Geometry: final body of the model. Coordinates: model frame, mm. Give positions to 0.01 mm unless a question says otherwise; leave off trailing zeros. Write each loop counter-clockwise with the first axis right and the second up, starting at its lowest first coordinate (ties: lowest second). Pieces come first, ordered by that corner, then holes. Notation, with made-up numbers: (-8, -37) - (28, -37) arc R28 ccw to (28, -10) - close; hole circle Ø11 at (-17, 50). An arc over 180 degrees is marked (long way). One line per question, with ' | ' between items. Start each with the question number.
```python
from build123d import *

# Parameters (mm, degrees)
F1_DEPTH = 127


with BuildPart() as f1:
    # F0 (on Front) → F1 (new body)
    with BuildSketch(Plane.XZ):
        with BuildLine():
            ThreePointArc((5.4872727498, -3.1956748535), (6.130525343, -1.6550404888), (6.35, 0))
            ThreePointArc((6.35, 0), (6.136710925, 1.6319555825), (5.5111719612, 3.1542802054))
            ThreePointArc((5.5111719612, 3.1542802054), (3.1956748226, 5.4872727678), (0.0238991973, 6.3499550257))
            ThreePointArc((0.0238991973, 6.3499550257), (-3.1542802223, 5.5111719515), (-5.4872727914, 3.195674782))
            ThreePointArc((-5.4872727914, 3.195674782), (-6.3499550258, 0.0238991699), (-5.5111719612, -3.1542802054))
            ThreePointArc((-5.5111719612, -3.1542802054), (-3.1956748226, -5.4872727678), (-0.0238991973, -6.3499550257))
            ThreePointArc((-0.0238991973, -6.3499550257), (3.1542801864, -5.511171972), (5.4872727498, -3.1956748535))
        make_face()
        with BuildLine():
            ThreePointArc((5.5111719612, 3.1542802054), (6.136710925, 1.6319555825), (6.35, 0))
            ThreePointArc((6.35, 0), (6.130525343, -1.6550404888), (5.4872727498, -3.1956748535))
            Line((5.4872727498, -3.1956748535), (7.3322964871, -0.027596355))
            Line((7.3322964871, -0.027596355), (5.5111719612, 3.1542802054))
        make_face()
        with BuildLine():
            ThreePointArc((0.0238991973, 6.3499550257), (3.1956748226, 5.4872727678), (5.5111719612, 3.1542802054))
            Line((5.5111719612, 3.1542802054), (3.690047388, 6.3361568484))
            Line((3.690047388, 6.3361568484), (0.0238991973, 6.3499550257))
        make_face()
        with BuildLine():
            Line((3.6422490991, -6.3637532034), (5.4872727498, -3.1956748535))
            ThreePointArc((5.4872727498, -3.1956748535), (3.1542801864, -5.511171972), (-0.0238991973, -6.3499550257))
            Line((-0.0238991973, -6.3499550257), (3.6422490991, -6.3637532034))
        make_face()
        with BuildLine():
            ThreePointArc((-5.4872727914, 3.195674782), (-3.1542802223, 5.5111719515), (0.0238991973, 6.3499550257))
            Line((0.0238991973, 6.3499550257), (-3.6422490991, 6.3637532034))
            Line((-3.6422490991, 6.3637532034), (-5.4872727914, 3.195674782))
        make_face()
        with BuildLine():
            Line((-3.690047388, -6.3361568484), (-0.0238991973, -6.3499550257))
            ThreePointArc((-0.0238991973, -6.3499550257), (-3.1956748226, -5.4872727678), (-5.5111719612, -3.1542802054))
            Line((-5.5111719612, -3.1542802054), (-3.690047388, -6.3361568484))
        make_face()
        with BuildLine():
            ThreePointArc((-5.5111719612, -3.1542802054), (-6.3499550258, 0.0238991699), (-5.4872727914, 3.195674782))
            Line((-5.4872727914, 3.195674782), (-7.3322964871, 0.027596355))
            Line((-7.3322964871, 0.027596355), (-5.5111719612, -3.1542802054))
        make_face()
    extrude(amount=F1_DEPTH)


solid = f1.part
```
1) Section B-B, the plane z = 5.25. Output: boundary loops of the cut face in (x, y).
2) Section A-A, the plane y = -53. Output: boundary loops of the cut face in (x, z).
3) First-contact query: pin 1 Ø4 at (x, y) = (1, -20.5) entering from +Z; pin 2 Ø1.5 at (y, z) = (-20, -3) entering from +X; pin 3 Ø2 at (y, z) = (-22, 0.5) entering from -X. Flat tips, straight axial feed; report the tip coordinate or a pass-through.
4) Section C-C, the plane z = -5. Output: boundary loops of the cut face in (x, y), plus the area to 3 significant figures.
5) Line query: L1, parallel to Z at x = -1, y = -103; L2, parallel to X at y = -24, z = 1.75; L3, parallel to Z at x = 2, y = -42. Output: solid intervals per line, ascending.
Answer key:
1) outline: (-4.29, -127) - (4.31, -127) - (4.31, 0) - (-4.29, 0) - close
2) outline: (-7.33, 0.03) - (-3.69, -6.34) - (3.64, -6.36) - (7.33, -0.03) - (3.69, 6.34) - (-3.64, 6.36) - close
3) pin 1: z = 6.35 | pin 2: x = 6.04 | pin 3: x = -7.33
4) outline: (-4.45, -127) - (4.44, -127) - (4.44, 0) - (-4.45, 0) - close | area: 1,130 mm^2
5) L1: -6.35 to 6.35 | L2: -6.33 to 6.31 | L3: -6.36 to 6.34
